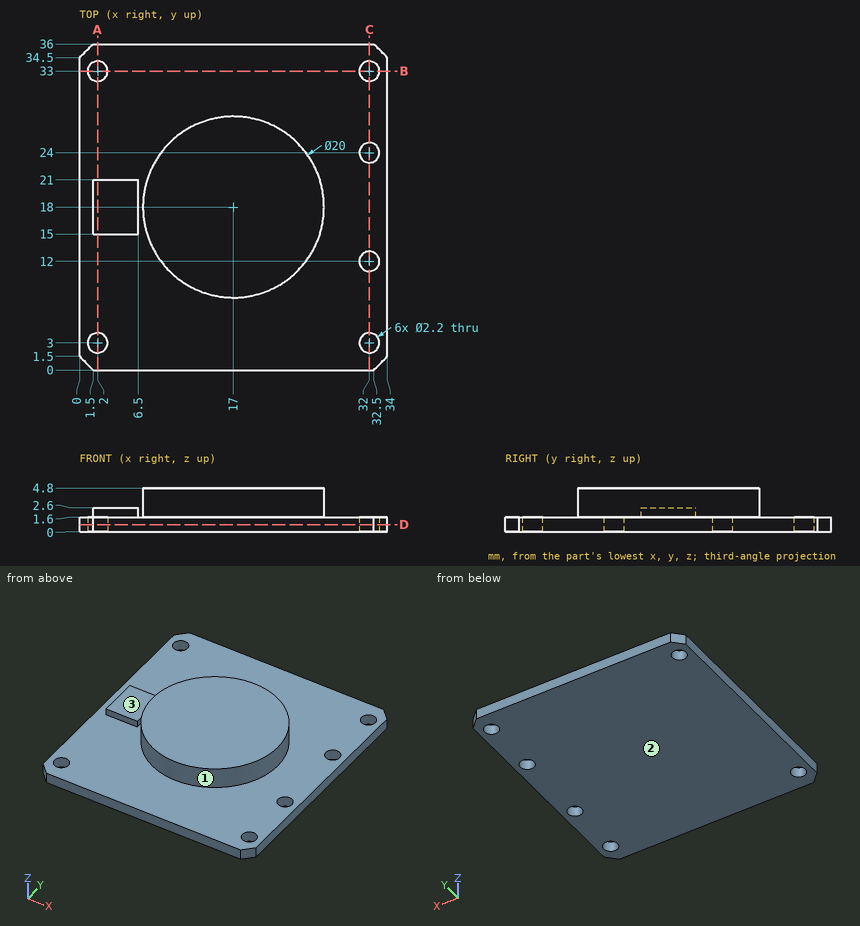
Verification items for this drawing (mm, ordinates from the low corner). A direction names the side the tool comes from. Coordinates: 2 decimals unless noted, no trailing zeros. Write each loop counter-clockwise with the first axis right and the second up, starting at its lowest first coordinate (ties: lowest second). Pieces come first, ordered by that corner, then holes. Notation, with made-up numbers: M -12.5,39 L -2.5,39 A7 ccw -2.5,48 Z; hole C -23,-39.5 d4. An arc over 180 degrees is marked long. One line per item, written item: value. Start each with the question number.
(1) Sectioned sample at D-D, the plane z = 0.75. Enter the section's corners in (x, y), and give its area (3 significant figures).
(2) Scan lines: line 1 along Y through (x, z) = (32, 1.1); line 2 along Y through (x, z) = (2, 1.25); line 3 along X through (y, z) = (12, 0.85). Record each from-to range of solid material in increasing order. Write a range as [from, to].
(3) Sectioned sample at B-B, the plane y = 33. Enter the section's corners in (x, z), and give its area (3 significant figures).
(4) Depth check by flat-ended pin: pin 1 (1.5 mm diameter, centred on x = 4, y = 17.5, fed in from +Z); pin 2 (1.3 mm diameter, centred on x = 32, y = 3, fed in from -Z); pin 3 (1.5 mm diameter, centred on x = 22, y = 16.5, fed in from -Z); pin 4 (3 mm diameter, centred on x = 32, y = 12, fed in from +Z). Enter the tip coordinate at first touch or a pass-through.
(5) Sectioned sample at A-A, the plane x = 2. Enter the section's corners in (y, z), and give its area (3 significant figures).
(6) Sectioned sample at C-C, the plane x = 32. Enter the section's corners in (y, z).
(7) Tool access check on the marked faces 1, 2 and 3. Record the directions out of +Z, -Z, +X, -X, +Y, -Y that give a thin tool (end or side, any length) a straight path to the whole face; none if there is none.
Filled sheet:
1. outline: M 0,1.5 L 1.5,0 L 32.5,0 L 34,1.5 L 34,34.5 L 32.5,36 L 1.5,36 L 0,34.5 Z; hole C 2,3 d2.2; hole C 2,33 d2.2; hole C 32,3 d2.2; hole C 32,12 d2.2; hole C 32,24 d2.2; hole C 32,33 d2.2
1. area: 1,200 mm²
2. line 1: [0, 1.9], [4.1, 10.9], [13.1, 22.9], [25.1, 31.9], [34.1, 36]
2. line 2: [0, 1.9], [4.1, 31.9], [34.1, 36]
2. line 3: [0, 30.9], [33.1, 34]
3. outline: M 0,0 L 0.9,0 L 0.9,1.6 L 0,1.6 Z; M 3.1,0 L 30.9,0 L 30.9,1.6 L 3.1,1.6 Z; M 33.1,0 L 34,0 L 34,1.6 L 33.1,1.6 Z
3. area: 47.4 mm²
4. pin 1: z = 2.6
4. pin 2: through
4. pin 3: z = 0
4. pin 4: z = 1.6
5. outline: M 0,0 L 1.9,0 L 1.9,1.6 L 0,1.6 Z; M 4.1,0 L 31.9,0 L 31.9,1.6 L 21,1.6 L 21,2.6 L 15,2.6 L 15,1.6 L 4.1,1.6 Z; M 34.1,0 L 36,0 L 36,1.6 L 34.1,1.6 Z
5. area: 56.6 mm²
6. outline: M 0,0 L 1.9,0 L 1.9,1.6 L 0,1.6 Z; M 4.1,0 L 10.9,0 L 10.9,1.6 L 4.1,1.6 Z; M 13.1,0 L 22.9,0 L 22.9,1.6 L 13.1,1.6 Z; M 25.1,0 L 31.9,0 L 31.9,1.6 L 25.1,1.6 Z; M 34.1,0 L 36,0 L 36,1.6 L 34.1,1.6 Z
7. face 1: +Z
7. face 2: -Z, +X, -X, +Y, -Y
7. face 3: +Z, -X, +Y, -Y
